The listing builds one solid part. Answer for the finished solid, in the listing's coordinates (mm). Face numbers are marked on the shaded views. A direction names the side the tool comes from. Give positions to 0.01 mm unless a question says otherwise; leave off trailing zeros. Loops run counter-clockwise (first coordinate to the right, second up) from the corner with the lowest first, then second, coordinate; pieces in that order, holes last.
Item 1: Consider line 1 along Y through (x, z) = (-245, 51); line 2 along Z through (x, y) = (-224, -265); line 3 along Y through (x, z) = (-176, 8.5). Determine where each line is inside the solid, lowest interval first.
Item 2: Section D-D, the plane y = -251.5 is taken. Give the vertices of the cut face in (x, z).
Item 3: Section A-A, the plane z = 32 is taken. Give the vertices of the cut face in (x, y).
Item 4: A tool of negligible diameter and unlimited length cuts with its end or side. For the marked faces 1 and 2, from which of +Z, -Z, +X, -X, +Y, -Y can it reach the whole face along a straight path? Write none if from no direction.
Item 5: Section B-B, the plane x = -403.5 is taken. Give the vertices of the cut face in (y, z).
Item 6: Each of these flat-tipped pins is pushed along its axis until it touches: pin 1 Ø4 at (x, z) = (-202, 22.5) entering from +Y; pin 2 Ø4.5 at (y, z) = (-45, 10) entering from -X; pin 3 Ø3 at (x, y) = (-170, -587) entering from +Z; pin 4 Ø9 at (y, z) = (-734, 20) entering from -X. Where does it stop, or does it pass through?
Item 7: Section C-C, the plane x = -264 is taken. Give the vertices of the cut face in (y, z), and give its area (3 significant figures).
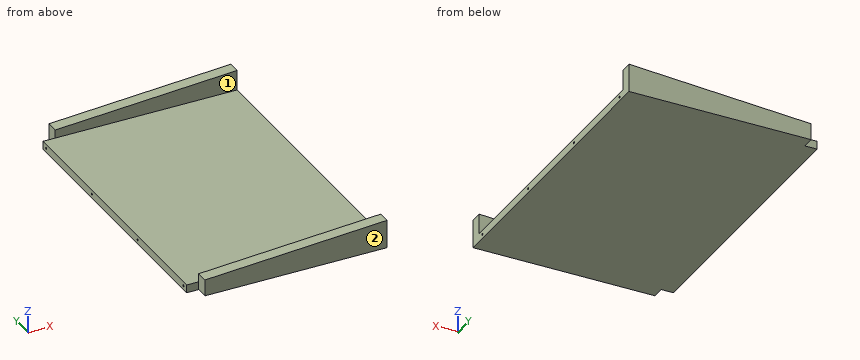
from build123d import *

# Parameters (mm, degrees)
F0_W      = 460
F0_H      = 750
F1_DEPTH  = 20
F3_D      = 5
F4_W      = 460
F4_H      = 30
F5_DEPTH  = 50
F7_DEPTH  = 750
F8_W      = 30
F8_H      = 40
F9_DEPTH  = 10
F10_DEPTH = 25
F11_DEPTH = 20


with BuildPart() as f1:
    # F0 (on Top) → F1 (new body)
    with BuildSketch(Plane.XY):
        with Locations((-230, -375)):
            Rectangle(F0_W, F0_H)
    extrude(amount=F1_DEPTH)

    # F3 (through all)
    with Locations(Plane.YZ):
        with Locations((-705, 10), (-485, 10), (-265, 10), (-45, 10)):
            Hole(F3_D / 2)

    # F4 (on face) → F5 (join)
    with BuildSketch(Plane.XY.offset(20)):
        with Locations((-230, -735)):
            Rectangle(F4_W, F4_H)
        with Locations((-230, -15)):
            Rectangle(F4_W, F4_H)
    extrude(amount=F5_DEPTH)

    # F6 (on face) → F7 (cut)
    with BuildSketch(Plane(origin=(0, 0, 0), x_dir=(-1, 0, 0), z_dir=(0, 1, 0))):
        Polygon((0, 70), (460, 40), (460, 70), align=None)
    extrude(amount=-F7_DEPTH, mode=Mode.SUBTRACT)

    # F8 (on face) → F9 (cut)
    with BuildSketch(Plane(origin=(-460, 0, 0), x_dir=(0, -1, 0), z_dir=(-1, 0, 0))):
        with Locations((15, 20)):
            Rectangle(F8_W, F8_H)
        with Locations((735, 20)):
            Rectangle(F8_W, F8_H)
    extrude(amount=-F9_DEPTH, mode=Mode.SUBTRACT)

    # F10 (cut): faces of the model
    f10_faces = [f1.faces().sort_by_distance(p)[0] for p in [
        (-455, -15, 40),
        (-455, -735, 40),
    ]]
    extrude(f10_faces, amount=-F10_DEPTH, mode=Mode.SUBTRACT)

    # F11 (add): a face of the model
    f11_faces = [f1.faces().sort_by_distance(p)[0] for p in [
        (-460, -375, 10),
    ]]
    extrude(f11_faces, amount=F11_DEPTH)


solid = f1.part
Worked answers:
1. line 1: y = -750 to -720, -30 to 0
1. line 2: z = 0 to 7.5, 12.5 to 20
1. line 3: y = -750 to -707, -703 to -487, -483 to -267, -263 to -47, -43 to 0
2. outline: (-480, 0) - (0, 0) - (0, 20) - (-480, 20) - close
3. outline: (-450, -750) - (0, -750) - (0, -720) - (-450, -720) - close; (-450, -30) - (0, -30) - (0, 0) - (-450, 0) - close
4. face 1: +Z, +X, -X
4. face 2: +Z, -Z, +X, -X, -Y
5. outline: (-750, 0) - (0, 0) - (0, 43.68) - (-30, 43.68) - (-30, 20) - (-720, 20) - (-720, 43.68) - (-750, 43.68) - close; hole circle Ø5 at (-705, 10); hole circle Ø5 at (-485, 10); hole circle Ø5 at (-265, 10); hole circle Ø5 at (-45, 10)
6. pin 1: stops at y = 0
6. pin 2: passes through
6. pin 3: stops at z = 20
6. pin 4: stops at x = -450
7. outline: (-750, 0) - (0, 0) - (0, 52.78) - (-30, 52.78) - (-30, 20) - (-720, 20) - (-720, 52.78) - (-750, 52.78) - close; hole circle Ø5 at (-705, 10); hole circle Ø5 at (-485, 10); hole circle Ø5 at (-265, 10); hole circle Ø5 at (-45, 10)
7. area: 16,900 mm2
